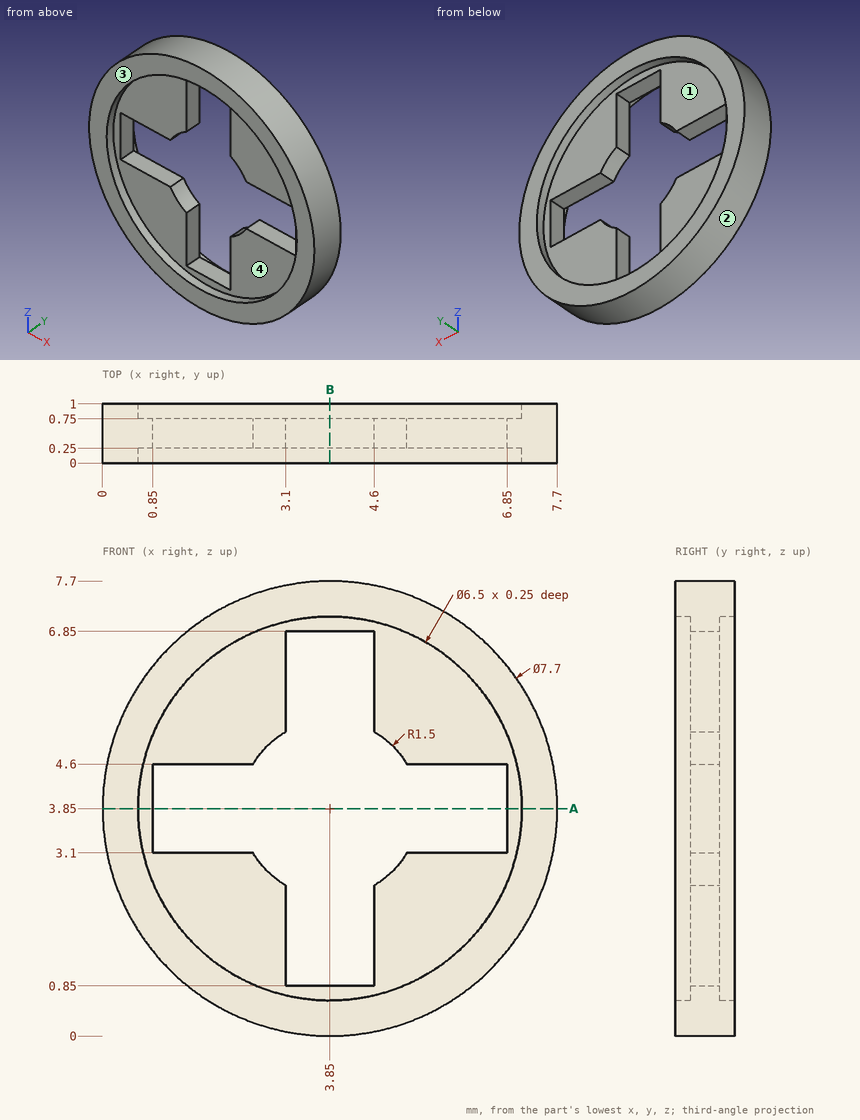
Geometry check sheet. Reference: drawing and pictorial views, mm from the part's lowest x, y, z. Round coordinates to 2 decimals unless told otherwise and drop trailing zeros. Order: outer loops, then holes, each group sorted by start corner. A loop starts at its lowest first (then second) coordinate and runs counter-clockwise, first axis right, second up. Notation, with made-up numbers: (-0.5, 49) - (43.5, 49) arc R30 cw to (43.5, 73) - close; hole circle Ø4 at (33.5, 57.5). An arc over 180 degrees is marked (long way). Use a Markdown table: item, result. Add a question column.
1) Thickness scan on line 1 along Z through (x, y) = (3.85, 0.85); line 2 along X through (y, z) = (0.9, 6); line 3 along X through (y, z) = (0.45, 4.5). Record the ranges inside material, lowest first.
2) Gauge pin test, flat ends, axial feed: P1, Ø3, axis at x = 2.5, z = 4, coming from the -Y side; P2, Ø2, axis at x = 5, z = 4, coming from the +Y side. Record the tip position at first contact, or that the pin passes through.
3) Mould release check, pull along X, two halves, no side actions. Record for the marked faces 1, 2, 3 and 4: released by +X, released by -X, zero draft, split by the parting line, or undercut.
4) Section check B-B (x = 3.85). Record the cut outline in (y, z), then the cut area to 3 significant figures.
5) Section check A-A (z = 3.85). Record the cut outline in (x, y), then the cut area to 3 significant figures.
Established:
| question | item | result |
|---|---|---|
| 1 | line 1 | 0 to 0.6, 7.1 to 7.7 |
| 1 | line 2 | 0.66 to 1.41, 6.29 to 7.04 |
| 1 | line 3 | 0.06 to 0.85, 6.85 to 7.64 |
| 2 | P1 | y = 0.25 |
| 2 | P2 | y = 0.75 |
| 3 | face 1 | undercut |
| 3 | face 2 | split by the parting line |
| 3 | face 3 | zero draft |
| 3 | face 4 | undercut |
| 4 | outline | (0, 0) - (1, 0) - (1, 0.6) - (0.75, 0.6) - (0.75, 0.85) - (0.25, 0.85) - (0.25, 0.6) - (0, 0.6) - close; (0, 7.1) - (0.25, 7.1) - (0.25, 6.85) - (0.75, 6.85) - (0.75, 7.1) - (1, 7.1) - (1, 7.7) - (0, 7.7) - close |
| 4 | area | 1.45 mm2 |
| 5 | outline | (0, 0) - (0.6, 0) - (0.6, 0.25) - (0.85, 0.25) - (0.85, 0.75) - (0.6, 0.75) - (0.6, 1) - (0, 1) - close; (6.85, 0.25) - (7.1, 0.25) - (7.1, 0) - (7.7, 0) - (7.7, 1) - (7.1, 1) - (7.1, 0.75) - (6.85, 0.75) - close |
| 5 | area | 1.45 mm2 |
